Part print with two shaded views. Sizes in mm from the minimum x, y, z corner. A direction names the side the tool comes from. Coordinates: 2 decimals unless noted, no trailing zeros. Loops run counter-clockwise (first coordinate to the right, second up) from the corner with the lowest first, then second, coordinate; pieces in that order, holes last.
(1) Flat gauge pins, fed straight in: P1, Ø1, axis at y = 5, z = 2.5, coming from the +X side; P2, Ø0.8, axis at x = 3, z = 3, coming from the +Y side (1 decimal); P3, Ø1, axis at x = 4.5, z = 0.5, coming from the +Y side. Where does each tip first touch, or does it go through?
(2) Slice it at A-A (x = 3.81). Give the cut face in (y, z) (1 decimal).
(3) Wall check: L1, parallel to Y at x = 3.81, z = 1.4; L2, parallel to Z at x = 6, y = 26; L3, parallel to X at y = 9.5, z = 1.55. Give the ranges that are in metal, low to high.
(4) Slice it at D-D (y = 19.25). Give the cut face in (x, z).
(5) Tool access for the marked faces 1 and 2: list every direction of +Z, -Z, +X, -X, +Y, -Y with a clear straight run to the whole face (end or side of a thin tool).
(6) Two-plate mould, pull along Y, no slides. Class the marked faces 3, 4 and 5: pulls with the +Y half, pulls with the -Y half, needs draft (parallel to the pull), parting line crosses it, or undercut.
(7) Slice it at B-B (y = 23.25). Give the cut face in (x, z).
(8) Slice it at C-C (z = 1.35). Give the cut face in (x, y) (1 decimal).
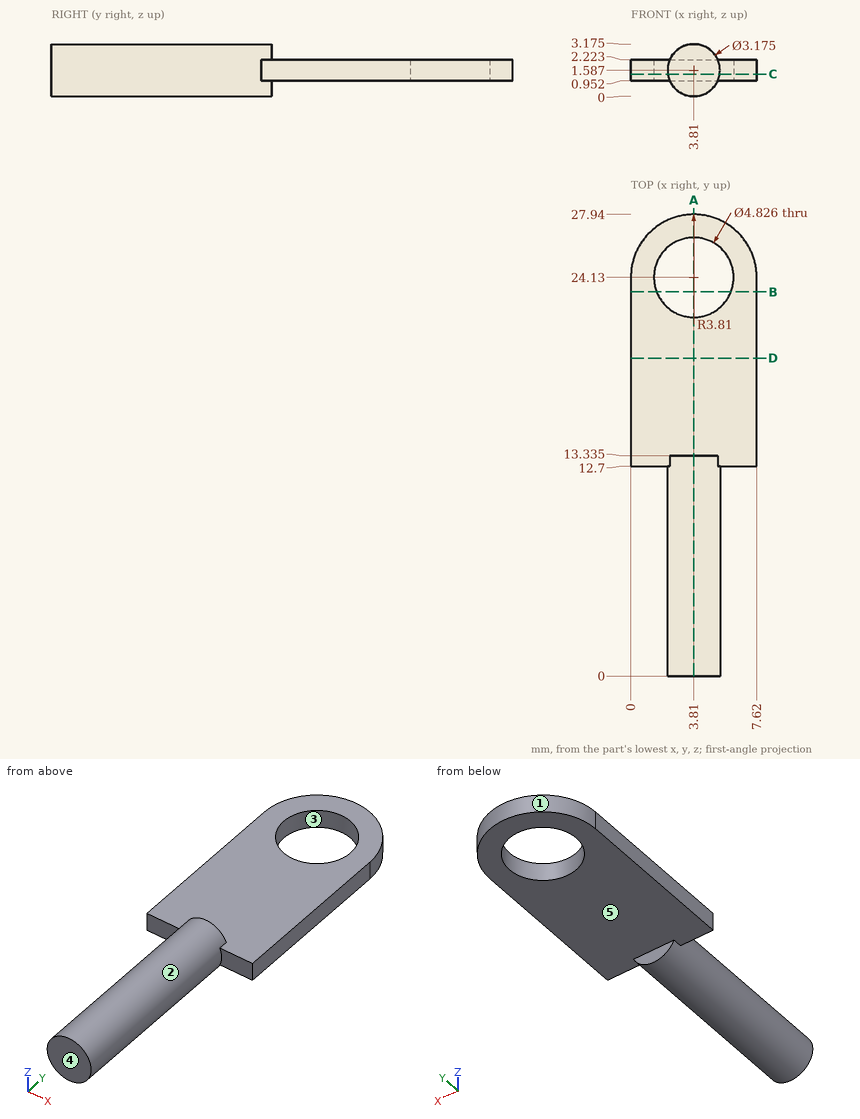
Response values:
1. P1: stops at x = 5.34
1. P2: stops at y = 13.3
1. P3: stops at y = 27.91
2. outline: (0, 0) - (13.3, 0) - (13.3, 1) - (21.7, 1) - (21.7, 2.2) - (13.3, 2.2) - (13.3, 3.2) - (0, 3.2) - close; (26.5, 1) - (27.9, 1) - (27.9, 2.2) - (26.5, 2.2) - close
3. L1: y = 0 to 21.72, 26.54 to 27.94
3. L2: z = 0.95 to 2.22
3. L3: x = 2.22 to 5.4
4. outline: (0, 0.95) - (7.62, 0.95) - (7.62, 2.22) - (0, 2.22) - close
5. face 1: +Z, -Z, +Y
5. face 2: -Y
6. face 3: undercut
6. face 4: pulls with the -Y half
6. face 5: needs draft
7. outline: (0, 0.95) - (1.56, 0.95) - (1.56, 2.22) - (0, 2.22) - close; (6.06, 0.95) - (7.62, 0.95) - (7.62, 2.22) - (6.06, 2.22) - close
8. outline: (0, 12.7) - (2.2, 12.7) - (2.2, 0) - (5.4, 0) - (5.4, 12.7) - (7.6, 12.7) - (7.6, 24.1) arc R3.8 ccw to (0, 24.1) - close; hole circle Ø4.8 at (3.8, 24.1)
